from build123d import *

# Parameters (mm, degrees)
ESQUISSE1_R             = 21.5
ESQUISSE1_R_2           = 11.25
BOSS_EXTRU_1_DEPTH      = 12
ESQUISSE2_R             = 2.5
ENL_V_MAT_EXTRU_1_DEPTH = 33.687918257
ESQUISSE4_R             = 3.75
ENL_V_MAT_EXTRU_2_DEPTH = 5
BOSS_EXTRU_2_START      = -8
ESQUISSE5_R             = 11.25
BOSS_EXTRU_2_DEPTH      = 8
ESQUISSE6_R             = 5
ENL_V_MAT_EXTRU_3_DEPTH = 50
ESQUISSE7_R             = 1.75
ENL_V_MAT_EXTRU_4_DEPTH = 11
ENL_V_MAT_EXTRU_5_DEPTH = 3


with BuildPart() as part:
    # Esquisse1 → Boss.-Extru.1 (new body)
    with BuildSketch(Plane.XY):
        Circle(ESQUISSE1_R)
        Circle(ESQUISSE1_R_2, mode=Mode.SUBTRACT)
    extrude(amount=BOSS_EXTRU_1_DEPTH)

    # Esquisse2 → Enlèv. mat.-Extru.1 (cut, through all)
    with BuildSketch(Plane.XY.offset(12)):
        with Locations((-14.713385832, 6.286197369)):
            Circle(ESQUISSE2_R)
        with Locations((6.28955657, 14.711950182)):
            Circle(ESQUISSE2_R)
        with Locations((14.713385832, -6.286197369)):
            Circle(ESQUISSE2_R)
        with Locations((-6.28955657, -14.711950182)):
            Circle(ESQUISSE2_R)
    extrude(amount=-ENL_V_MAT_EXTRU_1_DEPTH, mode=Mode.SUBTRACT)

    # Esquisse4 → Enlèv. mat.-Extru.2 (cut)
    with BuildSketch(Plane.XY.offset(12)):
        with Locations((-6.28955657, -14.711950182)):
            Circle(ESQUISSE4_R)
        with Locations((14.713385832, -6.286197369)):
            Circle(ESQUISSE4_R)
        with Locations((6.28955657, 14.711950182)):
            Circle(ESQUISSE4_R)
        with Locations((-14.713385832, 6.286197369)):
            Circle(ESQUISSE4_R)
    extrude(amount=-ENL_V_MAT_EXTRU_2_DEPTH, mode=Mode.SUBTRACT)

    # Esquisse5 → Boss.-Extru.2 (add)
    with BuildSketch(Plane.XY.offset(12).offset(BOSS_EXTRU_2_START)):
        Circle(ESQUISSE5_R)
    extrude(amount=BOSS_EXTRU_2_DEPTH)

    # Esquisse6 → Enlèv. mat.-Extru.3 (cut)
    with BuildSketch(Plane(origin=(0, 0, 4), x_dir=(-1, 0, 0), z_dir=(0, 0, -1))):
        Circle(ESQUISSE6_R)
    extrude(amount=-ENL_V_MAT_EXTRU_3_DEPTH, mode=Mode.SUBTRACT)

    # Esquisse7 → Enlèv. mat.-Extru.4 (cut)
    with BuildSketch(Plane(origin=(0, 0, 4), x_dir=(-1, 0, 0), z_dir=(0, 0, -1))):
        with Locations((7.420247562, -2.989970922)):
            Circle(ESQUISSE7_R)
        with Locations((-2.965758016, -7.429958236)):
            Circle(ESQUISSE7_R)
        with Locations((-7.27947207, 3.31802447)):
            Circle(ESQUISSE7_R)
        with Locations((3.367275567, 7.256821292)):
            Circle(ESQUISSE7_R)
    extrude(amount=-ENL_V_MAT_EXTRU_4_DEPTH, mode=Mode.SUBTRACT)

    # Esquisse8 → Enlèv. mat.-Extru.5 (cut)
    with BuildSketch(Plane.XY.offset(12)):
        Polygon((-6.817345267, 7.56830012), (-5.362058995, 4.4247127), (-1.911989294, 4.113233872), (0.082794134, 6.945342463), (-1.372492138, 10.088929883), (-4.822561839, 10.400408711), align=None)
        Polygon((7.630709315, 6.764273503), (4.470551482, 5.345329364), (4.119314237, 1.899080331), (6.928234824, -0.128224563), (10.088392657, 1.290719576), (10.439629903, 4.736968609), align=None)
        Polygon((6.351992849, -8.160309971), (5.291378589, -4.862568715), (1.905143756, -4.13221698), (-0.420476817, -6.699606501), (0.640137444, -9.997347757), (4.026372276, -10.727699492), align=None)
        Polygon((-6.701502779, 0.398746525), (-9.995590566, -0.673160957), (-10.71433535, -4.061878404), (-8.138992346, -6.378688369), (-4.844904559, -5.306780887), (-4.126159775, -1.91806344), align=None)
    extrude(amount=-ENL_V_MAT_EXTRU_5_DEPTH, mode=Mode.SUBTRACT)


solid = part.part
Part model, mm, in its own coordinate system. A direction names the side the tool comes from. Give positions to 0.01 mm unless a question says otherwise; leave off trailing zeros. Loops run counter-clockwise (first coordinate to the right, second up) from the corner with the lowest first, then second, coordinate; pieces in that order, holes last.
(1) Pull direction X, two halves, no side cores. Call faces 3 (the cylindrical face through (5.19, -9.98, 1.97)), 4 (the cylindrical face through (-2.799, 21.317, 5.916)): pulls with the +X half, pulls with the -X half, needs draft (parallel to the pull), parting line crosses it, or undercut.
Return value:
face 3: undercut
face 4: parting line crosses it
(2) Band-saw the part on B-B (x = -15). Write the cut outline in (y, z), and give its area (3 significant figures).
Return value:
outline: (-15.4, 0) - (3.8, 0) - (3.8, 7) - (2.55, 7) - (2.55, 12) - (-15.4, 12) - close; (8.77, 0) - (15.4, 0) - (15.4, 12) - (10.03, 12) - (10.03, 7) - (8.77, 7) - close
area: 298 mm2
(3) Drill centre lines: line 1 along X through (y, z) = (8.5, 6); line 2 along X through (y, z) = (7.5, 9.25); line 3 along Y through (x, z) = (5, 1.5). Where is each one in solid material? Low to high.
Return value:
line 1: x = -19.75 to -15.87, -13.55 to -4.6, -2.14 to 19.75
line 2: x = -20.15 to -18.26, -11.17 to -6.79, -0.17 to 20.15
line 3: y = -20.91 to -10.08, 10.08 to 12.57, 16.85 to 20.91
(4) Band-saw the part on C-C (z = 2). Write the cut outline in (x, y), and give its area (3 significant figures).
Return value:
outline: circle Ø43 at (0, 0); hole circle Ø5 at (-14.71, 6.29); hole circle Ø22.5 at (0, 0); hole circle Ø5 at (-6.29, -14.71); hole circle Ø5 at (6.29, 14.71); hole circle Ø5 at (14.71, -6.29)
area: 976 mm2
(5) 3-axis set-ups, long thin cutter, end or side, ignore diameter. For faces 1 (the flat face through (6.073, 6.065, 10.521)), 2 (the cylindrical face through (3.194, -5.695, 6.465)): which of +Z, -Z, +X, -X, +Y, -Y reach the whole face in a straight line?
Return value:
face 1: +Z
face 2: +Z, -Z
(6) Band-saw the part on A-A (z = 7.75). Count the separate pieces of the cut face and the enclosed holes in it, and give its area (3 significant figures).
Return value:
separate pieces: 1
enclosed holes: 9
area: 1,160 mm2
(7) Pin check, flat tips, straight feed: pin 1 (1 mm diameter, centred on x = 7.5, z = 8.5, fed in from +Y); pin 2 (4 mm diameter, centred on x = -7.42, y = -2.99, fed in from +Z); pin 3 (5.5 mm diameter, centred on x = 2.97, y = -7.43, fed in from -Z); pin 4 (6 mm diameter, centred on x = 0, y = 0, fed in from +Z). Stop position of each tip, or through.
Return value:
pin 1: stops at y = 20.33
pin 2: stops at z = 9
pin 3: stops at z = 4
pin 4: passes through
